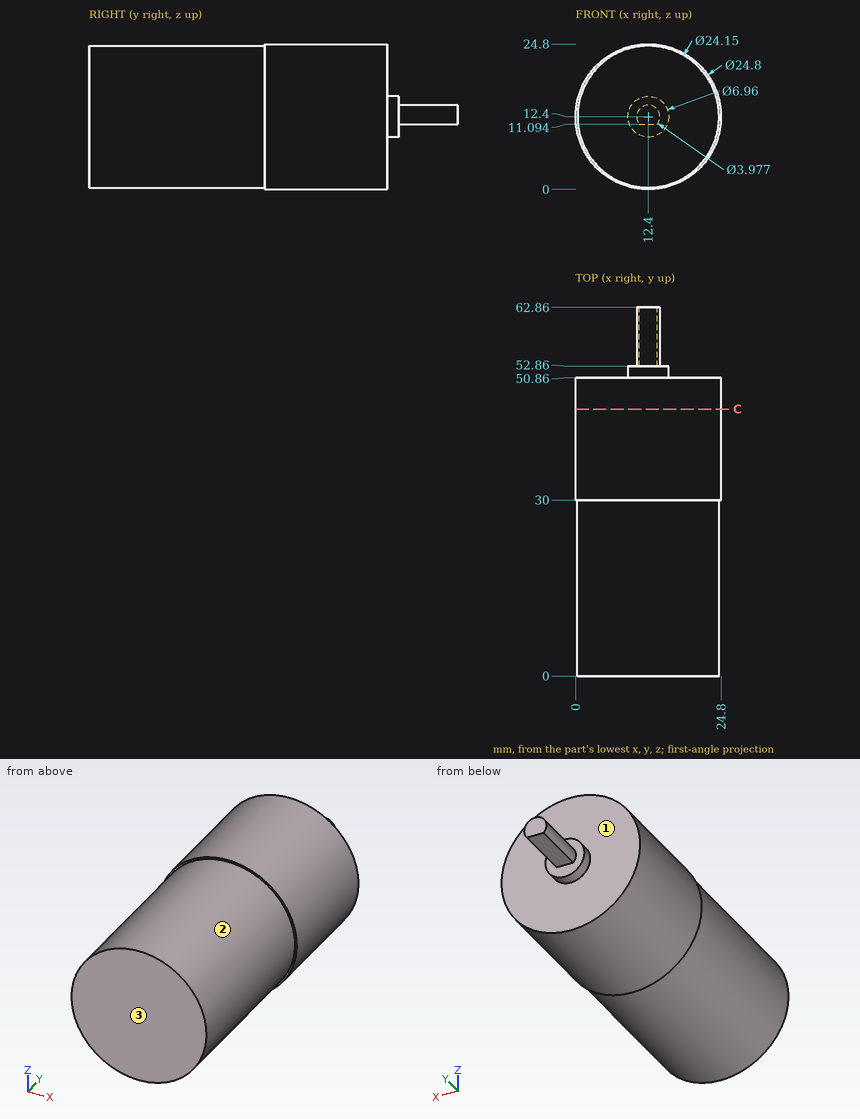
Study the drawing (mm; zero at the part's minimum x, y, z) and answer. Coordinates: 2 decimals unless noted, no trailing zeros. Loops run counter-clockwise (first coordinate to the right, second up) from the corner with the lowest first, then second, coordinate; pieces in that order, holes last. Notation, with made-up numbers: (1, 83) -> (28, 83) arc R28 cw to (28, 103) -> close; hole circle Ø5 at (67.5, 57). An arc over 180 degrees is marked (long way). Answer in a Markdown table with one row per item. Add a question column.
1. Flat-ended cylindrical pins translate along their axes: P1, Ø1.5, axis at x = 12.5, y = 56.5, coming from the -Z side; P2, Ø1.5, axis at x = 9.5, y = 51, coming from the -Z side; P3, Ø1.5, axis at y = 27.5, z = 13, coming from the +X side (3 decimals). Find the tip coordinate at first contact, or state that the pin passes through.
2. Consider line 1 (Y direction, x = 6.25, z = 14.5); line 2 (X direction, y = 35, z = 13) (1 decimal); line 3 (X direction, y = 35.5, z = 23.5) (1 decimal). Determine where each line is inside the solid, lowest interval first. Write a range as [from, to].
3. The part is cut by section C-C, the plane y = 45.5. Write down the section's boundary in (x, z).
4. Determine the mould class of the marked faces 1, 2 and 3 for opening direction Y: +Y half, -Y half, draft (parallel to the pull), parting line (faces both ways), or undercut.
Answer below:
| question | item | result |
|---|---|---|
| 1 | P1 | z = 11.09 |
| 1 | P2 | z = 0.19 |
| 1 | P3 | x = 24.475 |
| 2 | line 1 | [0, 50.86] |
| 2 | line 2 | [0, 24.8] |
| 2 | line 3 | [6.9, 17.9] |
| 3 | outline | circle Ø24.8 at (12.4, 12.4) |
| 4 | face 1 | +Y half |
| 4 | face 2 | draft |
| 4 | face 3 | -Y half |
